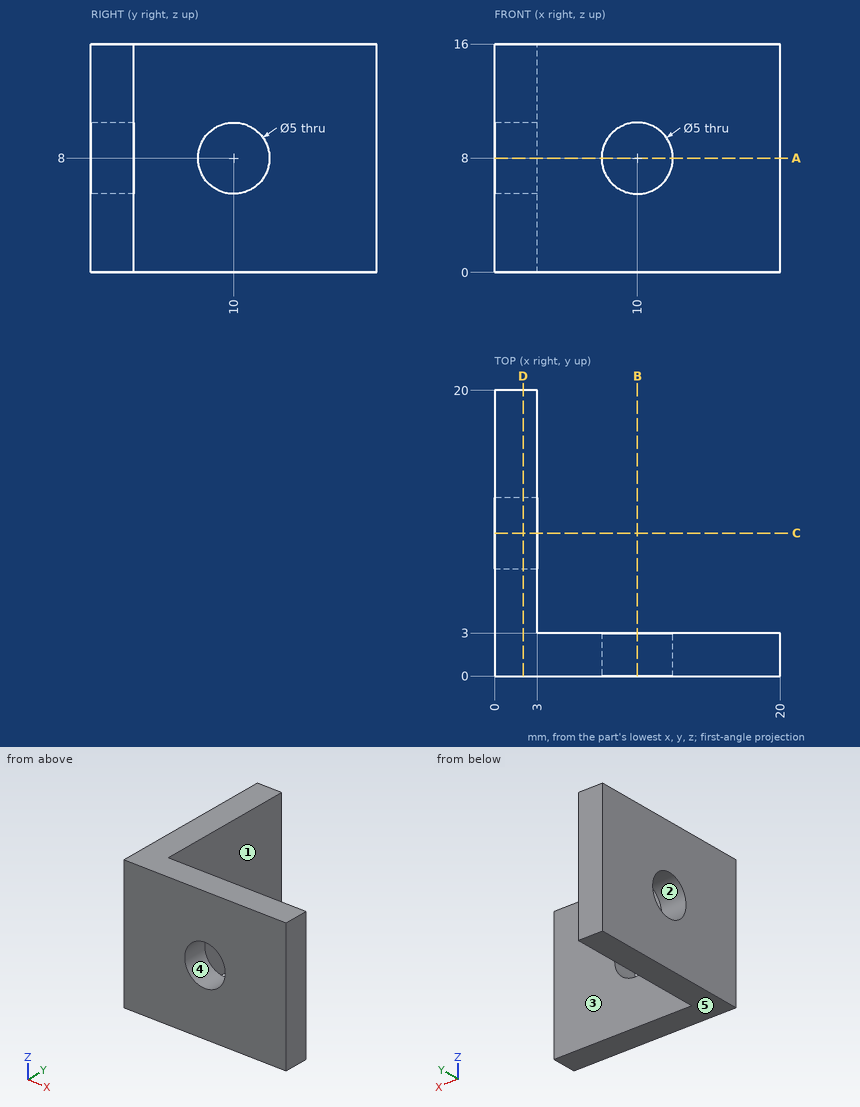
For this review, use the dimensioned drawing (mm, ordinates from the lowest corner) and the shaded views. A direction names the side the tool comes from. Coordinates: 2 decimals unless noted, no trailing zeros. Loops run counter-clockwise (first coordinate to the right, second up) from the corner with the lowest first, then second, coordinate; pieces in that order, holes last. Notation, with made-up numbers: (42.25, 13) - (63.25, 13) arc R16 cw to (63.25, 26) - close; hole circle Ø11 at (-23, -21.5). An arc over 180 degrees is marked (long way). Use CSV: the item, a comma, the result in double quotes. Start each with the question number.
1) Tool access review of the marked faces 1 and 2: name each direction out of +Z, -Z, +X, -X, +Y, -Y from which nothing blocks a thin tool from reaching the whole face with its end or side.
2) The part is to be moulded in two halves that separate along Z. For the marked faces 3, 4 and 5, say which applies: +Z half, -Z half, draft (parallel to the pull), parting line (faces both ways), or undercut.
3) Consider section B-B on x = 10. Write out the cut boundary in (y, z).
4) Consider section D-D on x = 2. Write out the cut boundary in (y, z), then the cut area to 3 significant figures.
5) Wall thickness on L1, parallel to Z at x = 10, y = 1.8; L2, parallel to Y at x = 9, z = 14: over which ranges is each line inside the solid? List them lowest first. Write a range as from..to.
6) For pin 1 Ø6.5 at (y, z) = (10, 8) entering from +X; pin 2 Ø4 at (x, z) = (7.5, 9) entering from +Y, all flat-tipped, find the tip position at first contact; note any pin that passes through.
7) Consider section A-A on z = 8. Write out the cut boundary in (x, y), then the cut area to 3 significant figures.
Geometry says:
1,face 1,"+Z, -Z, +X, +Y"
1,face 2,"+X, -X"
2,face 3,"draft"
2,face 4,"undercut"
2,face 5,"-Z half"
3,outline,"(0, 0) - (3, 0) - (3, 5.5) - (0, 5.5) - close; (0, 10.5) - (3, 10.5) - (3, 16) - (0, 16) - close"
4,outline,"(0, 0) - (20, 0) - (20, 16) - (0, 16) - close; hole circle Ø5 at (10, 8)"
4,area,"300 mm^2"
5,L1,"0..5.5, 10.5..16"
5,L2,"0..3"
6,pin 1,"x = 3"
6,pin 2,"y = 3"
7,outline,"(0, 0) - (7.5, 0) - (7.5, 3) - (3, 3) - (3, 7.5) - (0, 7.5) - close; (0, 12.5) - (3, 12.5) - (3, 20) - (0, 20) - close; (12.5, 0) - (20, 0) - (20, 3) - (12.5, 3) - close"
7,area,"81.0 mm^2"
